The drawing under review shows one solid part. Ordinate dimensions are in mm from its lowest x, y, z. Coordinates: 2 decimals unless noted, no trailing zeros. Write each loop counter-clockwise with the first axis right and the second up, starting at its lowest first coordinate (ties: lowest second). Pieces come first, ordered by that corner, then holes.
Q1. Add section B-B, the plane y = 28.5. Give the boundary of the cut face in (x, z), plus the area to 3 significant figures.
Q2. Add section A-A, the plane z = 3.9. Give the boundary of the cut face in (x, y), plus the area to 3 significant figures.
Q3. To check wall thickness, follow probe 1 along Y at (x, z) = (78, 3.6); probe 2 along X at (y, z) = (21, 3.15); probe 3 along X at (y, z) = (45, 2.1). State the ranges of each line that lie inside material, in increasing order.
Q4. Clearance check with flat-ended pins moving along their axes: pin 1 Ø2.5 at (y, z) = (45.5, 3.5) entering from +X; pin 2 Ø1.5 at (y, z) = (26, 2) entering from -X; pin 3 Ø2.5 at (x, z) = (82, 3.5) entering from -Y. State where each tip first meets the part, or that it passes through.
Q5. Add section C-C, the plane x = 79. Give the boundary of the cut face in (y, z), plus the area to 3 significant figures.
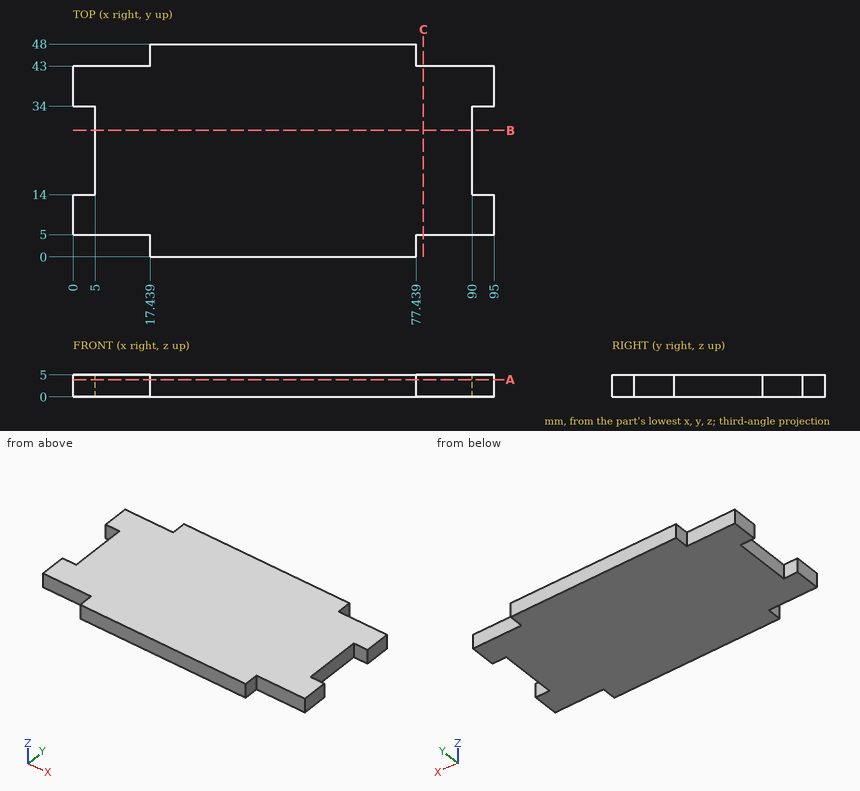
Here are the results:
1. outline: (5, 0) - (90, 0) - (90, 5) - (5, 5) - close
1. area: 425 mm2
2. outline: (0, 5) - (17.44, 5) - (17.44, 0) - (77.44, 0) - (77.44, 5) - (95, 5) - (95, 14) - (90, 14) - (90, 34) - (95, 34) - (95, 43) - (77.44, 43) - (77.44, 48) - (17.44, 48) - (17.44, 43) - (0, 43) - (0, 34) - (5, 34) - (5, 14) - (0, 14) - close
2. area: 4,010 mm2
3. probe 1: y = 5 to 43
3. probe 2: x = 5 to 90
3. probe 3: x = 17.44 to 77.44
4. pin 1: stops at x = 77.44
4. pin 2: stops at x = 5
4. pin 3: stops at y = 5
5. outline: (5, 0) - (43, 0) - (43, 5) - (5, 5) - close
5. area: 190 mm2
